Geometry check sheet. Reference: the model listing, model coordinates, mm. A direction names the side the tool comes from. Give positions to 0.01 mm unless a question says otherwise; leave off trailing zeros. Loops run counter-clockwise (first coordinate to the right, second up) from the corner with the lowest first, then second, coordinate; pieces in that order, holes last. Notation, with made-up numbers: (64.25, 73) -> (82.25, 73) arc R27 ccw to (82.25, 91) -> close; hole circle Ø9 at (-37, -36). An arc over 180 degrees is marked (long way). Answer in a Markdown table with one row per item. Add a question column.
```python
from build123d import *

# Parameters (mm, degrees)
BOSS_EXTRUDE1_DEPTH = 6.35


with BuildPart() as part:
    # Sketch1 → Boss-Extrude1 (new body)
    with BuildSketch(Plane(origin=(0, 0, 0), x_dir=(1, 0, 0), z_dir=(0, 1, 0))):
        with BuildLine():
            Line((50, -10), (50, -7.05))
            Line((50, -7.05), (47, -7.05))
            Line((47, -7.05), (47, -8.55))
            Line((47, -8.55), (43.7, -8.55))
            Line((43.7, -8.55), (43.7, -7.05))
            Line((43.7, -7.05), (38, -7.05))
            Line((38, -7.05), (38, -2.95))
            Line((38, -2.95), (43.7, -2.95))
            Line((43.7, -2.95), (43.7, -1.45))
            Line((43.7, -1.45), (47, -1.45))
            Line((47, -1.45), (47, -2.95))
            Line((47, -2.95), (50, -2.95))
            Line((50, -2.95), (50, 2.95))
            Line((50, 2.95), (47, 2.95))
            Line((47, 2.95), (47, 1.45))
            Line((47, 1.45), (43.7, 1.45))
            Line((43.7, 1.45), (43.7, 2.95))
            Line((43.7, 2.95), (38, 2.95))
            Line((38, 2.95), (38, 7.05))
            Line((38, 7.05), (43.7, 7.05))
            Line((43.7, 7.05), (43.7, 8.55))
            Line((43.7, 8.55), (47, 8.55))
            Line((47, 8.55), (47, 7.05))
            Line((47, 7.05), (50, 7.05))
            Line((50, 7.05), (50, 10))
            Line((50, 10), (25, 10))
            ThreePointArc((25, 10), (21.043842997, 9.646494123), (17.213036448, 8.59717729))
            ThreePointArc((17.213036448, 8.59717729), (13.403865442, 7.463896906), (9.477065544, 6.852054824))
            Line((9.477065544, 6.852054824), (-0.522934456, 5.977168189))
            ThreePointArc((-0.522934456, 5.977168189), (-6, 0), (-0.522934456, -5.977168189))
            Line((-0.522934456, -5.977168189), (9.477065544, -6.852054824))
            ThreePointArc((9.477065544, -6.852054824), (13.403865442, -7.463896906), (17.213036448, -8.59717729))
            ThreePointArc((17.213036448, -8.59717729), (21.043842997, -9.646494123), (25, -10))
            Line((25, -10), (50, -10))
        make_face()
        Polygon((0, 2.895), (-0.332133069, 2.629103958), (-0.719957223, 2.804048251), (-0.975530065, 2.463907688), (-1.394676887, 2.536907839), (-1.557630919, 2.143895035), (-1.981763872, 2.110364176), (-2.041860093, 1.689173573), (-2.444329344, 1.551218571), (-2.397791689, 1.128315123), (-2.753308615, 0.894604199), (-2.603061214, 0.496560484), (-2.889287379, 0.181778554), (-2.64477083, -0.166394877), (-2.843721591, -0.542468906), (-2.520299768, -0.818895035), (-2.619474317, -1.232631049), (-2.237469003, -1.419941007), (-2.230635838, -1.84534245), (-1.814049831, -1.931766863), (-1.701638305, -2.342104199), (-1.276647236, -2.322212702), (-1.06572058, -2.691702927), (-0.659028201, -2.566745377), (-0.362839711, -2.87217206), (0, -2.65), (0.362839711, -2.87217206), (0.659028201, -2.566745377), (1.06572058, -2.691702927), (1.276647236, -2.322212702), (1.701638305, -2.342104199), (1.814049831, -1.931766863), (2.230635838, -1.84534245), (2.237469003, -1.419941007), (2.619474317, -1.232631049), (2.520299768, -0.818895035), (2.843721591, -0.542468906), (2.64477083, -0.166394877), (2.889287379, 0.181778554), (2.603061214, 0.496560484), (2.753308615, 0.894604199), (2.397791689, 1.128315123), (2.444329344, 1.551218571), (2.041860093, 1.689173573), (1.981763872, 2.110364176), (1.557630919, 2.143895035), (1.394676887, 2.536907839), (0.975530065, 2.463907688), (0.719957223, 2.804048251), (0.332133069, 2.629103958), align=None, mode=Mode.SUBTRACT)
    extrude(amount=BOSS_EXTRUDE1_DEPTH)


solid = part.part
```
1. Gauge pin test, flat ends, axial feed: pin 1 Ø1.2 at (y, z) = (3, 4.5) entering from +X; pin 2 Ø12 at (x, z) = (44, -3) entering from -Y; pin 3 Ø0.5 at (y, z) = (2.5, -2) entering from -X. Record the tip position at first contact, or that the pin passes through.
2. Access from +Z, -Z, +X, -X, +Y, -Y to the whole of each face (thin tool, end or side, straight path). Record for faces 4 (the face through (45, 3, 1.45)), 5 (the face through (20.989, 3.131, 9.637)), 6 (the face through (38, 3, -5)).
3. Sectioned sample at B-B (z = -5). Enter the section's corners in (x, y), plus the area to 3 significant figures.
4. Release check for a two-part mould opening along X. For faces 1 (the face through (50, 3, 9)), 2 (the face through (45, 3, 8.55)), 3 (the face through (22, 0, 0)) record: released by +X, released by -X, zero draft, split by the parting line, or undercut.
5. Sectioned sample at A-A (x = 45). Enter the section's corners in (y, z).
6. Material ranges on L1, parallel to Z at x = 41, y = 5; L2, parallel to X at y = 0.5, z = 1.5; L3, parallel to X at y = 3.5, z = -0.25, recorded low to high. Write a range as from..to.
7. Sectioned sample at C-C (x = 16). Enter the section's corners in (y, z).
Response:
| question | item | result |
|---|---|---|
| 1 | pin 1 | stops at x = 38 |
| 1 | pin 2 | stops at y = 0 |
| 1 | pin 3 | stops at x = -5.74 |
| 2 | face 4 | +Y, -Y |
| 2 | face 5 | +Z, -X, +Y, -Y |
| 2 | face 6 | +X, +Y, -Y |
| 3 | outline | (-3.32, 0) -> (38, 0) -> (38, 6.35) -> (-3.32, 6.35) -> close |
| 3 | area | 262 mm2 |
| 4 | face 1 | released by +X |
| 4 | face 2 | undercut |
| 4 | face 3 | zero draft |
| 5 | outline | (0, -10) -> (6.35, -10) -> (6.35, -8.55) -> (0, -8.55) -> close; (0, -1.45) -> (6.35, -1.45) -> (6.35, 1.45) -> (0, 1.45) -> close; (0, 8.55) -> (6.35, 8.55) -> (6.35, 10) -> (0, 10) -> close |
| 6 | L1 | z = -10..-7.05, -2.95..2.95, 7.05..10 |
| 6 | L2 | x = -5.81..-2.24, 2.24..43.7, 47..50 |
| 6 | L3 | x = -5.99..-2.83, 2.83..50 |
| 7 | outline | (0, -8.18) -> (6.35, -8.18) -> (6.35, 8.18) -> (0, 8.18) -> close |
